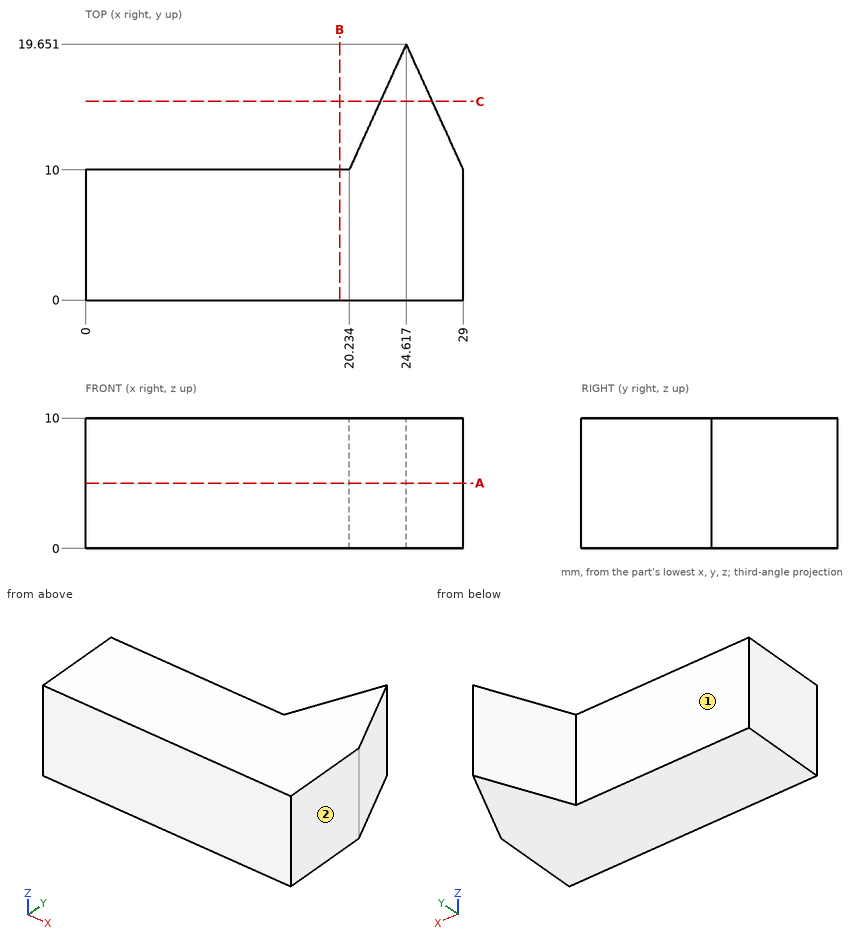
Answer from the drawing. Dimensions are ordinates in mm from the lowest x, y and z of the part. A direction names the side the tool comes from. Round coordinates to 2 decimals unless told otherwise and drop trailing zeros. Write each loop counter-clockwise with the first axis right and the second up, starting at its lowest first coordinate (ties: lowest second). Pieces come first, ordered by that corner, then holes. Notation, with made-up numbers: (26, 72) -> (59, 72) arc R28 ccw to (59, 104) -> close; hole circle Ø9 at (-20.75, 10.25). An arc over 180 degrees is marked (long way). Write each question's results on one line, items separated by ' | '.
1) The part is cut by section A-A (z = 5). Write down the section's boundary in (x, y), and give its area (3 significant figures).
Findings:
outline: (0, 0) -> (29, 0) -> (29, 10) -> (24.62, 19.65) -> (20.23, 10) -> (0, 10) -> close | area: 332 mm²
2) Flat-ended cylindrical pins translate along their axes: pin 1 (4 mm diameter, centred on x = 13.5, z = 2.5, fed in from +Y); pin 2 (1 mm diameter, centred on y = 12.5, z = 3.5, fed in from +X). Find the tip coordinate at first contact, or state that the pin passes through.
Findings:
pin 1: stops at y = 10 | pin 2: stops at x = 28.09
3) The part is cut by section C-C (y = 15.25). Write down the section's boundary in (x, z) (1 decimal).
Findings:
outline: (22.6, 0) -> (26.6, 0) -> (26.6, 10) -> (22.6, 10) -> close
4) The part is cut by section B-B (x = 19.5). Write down the section's boundary in (y, z).
Findings:
outline: (0, 0) -> (10, 0) -> (10, 10) -> (0, 10) -> close
5) Consider line 1 along Y through (x, z) = (16.5, 2.75); line 2 along X through (y, z) = (17, 7.25); line 3 along X through (y, z) = (12.75, 3.5). Determine where each line is inside the solid, lowest interval first. Write a range as [from, to].
Findings:
line 1: y = [0, 10] | line 2: x = [23.41, 25.82] | line 3: x = [21.48, 27.75]
6) Which of the six approach directions +Z, -Z, +X, -X, +Y, -Y give full straight-line access (tool end or side, diameter ignored) to the marked faces 1 and 2?
Findings:
face 1: +Z, -Z, -X, +Y | face 2: +Z, -Z, +X, +Y, -Y
